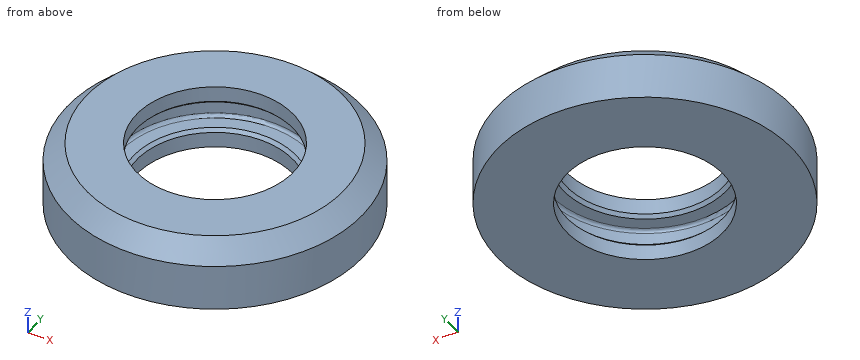
Autodesk Inventor part; units mm, degrees
ref_plane "YZ Plane" through (0, 0, 0) normal (1, 0, 0) x (0, 1, 0)
ref_plane "XZ Plane" through (0, 0, 0) normal (0, 1, 0) x (-1, 0, 0)
ref_plane "XY Plane" through (0, 0, 0) normal (0, 0, 1) x (1, 0, 0)
sketch "草圖1" plane through (0, 0, 0) normal (0, 0, 1) x (1, 0, 0)
  circle A0 centre (0, 0) radius 23.5
  dimension "d0" = 47
extrude "擠出1" add sketch "草圖1" along normal blind 10.4
chamfer "倒角1" distance 3 angle 45 1 edges at (-23.5, 0, 10.4)
sketch "草圖3" plane through (0, 0, 10.4) normal (0, 0, 1) x (1, 0, 0)
  circle A0 centre (0, 0) radius 20.5
hole "孔1" at (0, 0, 10.4) direction (0, 0, -1) diameter 25 end through all
sketch "草圖4" plane through (0, 0, 0) normal (0, 1, 0) x (-1, 0, 0)
  line L0 (0, 0) -> (0, 3)
  line L1 (-15.55, 7.4) -> (15.55, 7.4)
  line L2 (15.55, 7.4) -> (15.55, 3)
  line L3 (15.55, 3) -> (-15.55, 3)
  line L4 (-15.55, 3) -> (-15.55, 7.4)
  line L5 (0, 7.4) -> (0, 3)
  dimension "d13" = 3
  dimension "d14" = 31.1
  dimension "d15" = 4.4
revolve "迴轉1" cut sketch "草圖4" angle 360 about axis through (0, 0, 7.4) along (0, 0, -1) contours L1 L2 L3 L5
fillet "圓角1" radius 0.5 2 edges at (15.55, 0, 3) (15.55, 0, 7.4)
chamfer "倒角2" distance 0.5 angle 45 2 edges at (0, 12.5, 7.4) (0, 12.5, 3)
properties part number "機械油封墊片-KMB601PT-t10.4"
The listing builds one solid part. Answer for the finished solid, in the listing's coordinates (mm). Coordinates: 2 decimals unless noted, no trailing zeros. Order: outer loops, then holes, each group sorted by start corner. A loop starts at its lowest first (then second) coordinate and runs counter-clockwise, first axis right, second up. Notation, with made-up numbers: (75, 51.25) -> (89, 51.25) arc R16 ccw to (89, 55.25) -> close; hole circle Ø10 at (-1.75, 40). An arc over 180 degrees is marked (long way). Answer in a Markdown table with one row per item. Add a question column.
Item 1: Find the intervals of material crossed by L1, parallel to Y at x = 0, z = 0.6; L2, parallel to Z at x = 15, y = 0; L3, parallel to Y at x = 0, z = 5, in increasing order. Write a range as from..to.
Item 2: Find section C-C (z = 6). Write down the section's boundary in (x, y), then the cut area to 3 significant figures.
Item 3: Find section A-A (x = 0). Write down the section's boundary in (y, z), then the cut area to 3 significant figures.
Item 4: Each of these flat-tipped pins is pushed along its axis until it touches: P1, Ø1, axis at y = 9, z = 5.5, coming from the +X side; P2, Ø2, axis at y = 13.5, z = 4.5, coming from the +X side; P3, Ø3, axis at x = 12, y = 1.5, coming from the -Z side; P4, Ø5, axis at y = 6, z = 5.5, coming from the +X side. Where does it stop, or does it pass through?
Result set:
| question | item | result |
|---|---|---|
| 1 | L1 | y = -23.5..-12.5, 12.5..23.5 |
| 1 | L2 | z = 0..3, 7.4..10.4 |
| 1 | L3 | y = -23.5..-15.55, 15.55..23.5 |
| 2 | outline | circle Ø47 at (0, 0); hole circle Ø31.1 at (0, 0) |
| 2 | area | 975 mm² |
| 3 | outline | (-23.5, 0) -> (-12.5, 0) -> (-12.5, 2.5) -> (-13, 3) -> (-15.05, 3) arc R0.5 cw to (-15.55, 3.5) -> (-15.55, 6.9) arc R0.5 cw to (-15.05, 7.4) -> (-13, 7.4) -> (-12.5, 7.9) -> (-12.5, 10.4) -> (-20.5, 10.4) -> (-23.5, 7.4) -> close; (12.5, 0) -> (23.5, 0) -> (23.5, 7.4) -> (20.5, 10.4) -> (12.5, 10.4) -> (12.5, 7.9) -> (13, 7.4) -> (15.05, 7.4) arc R0.5 cw to (15.55, 6.9) -> (15.55, 3.5) arc R0.5 cw to (15.05, 3) -> (13, 3) -> (12.5, 2.5) -> close |
| 3 | area | 193 mm² |
| 4 | P1 | stops at x = 21.91 |
| 4 | P2 | stops at x = 19.9 |
| 4 | P3 | stops at z = 0 |
| 4 | P4 | stops at x = 23.24 |
